```python
from build123d import *

# Parameters (mm, degrees)
F0_W     = 30
F0_H     = 60
F1_DEPTH = 5
F2_R     = 2.196128
F3_DEPTH = 3
F4_R     = 1.034036
F5_DEPTH = 1


with BuildPart() as f1:
    # F0 (on Front) → F1 (new body)
    with BuildSketch(Plane.XZ):
        with Locations((-16.133093, -22.920842)):
            Rectangle(F0_W, F0_H)
    extrude(amount=F1_DEPTH)

    # F2 (on face) → F3 (join)
    with BuildSketch(Plane.XZ.offset(5)):
        with Locations((-7.345827, -21.091014)):
            Circle(F2_R)
    extrude(amount=F3_DEPTH)

    # F4 (on face) → F5 (join)
    with BuildSketch(Plane.XZ.offset(8)):
        with Locations((-7.345827, -21.091014)):
            Circle(F4_R)
    extrude(amount=F5_DEPTH)


solid = f1.part
```
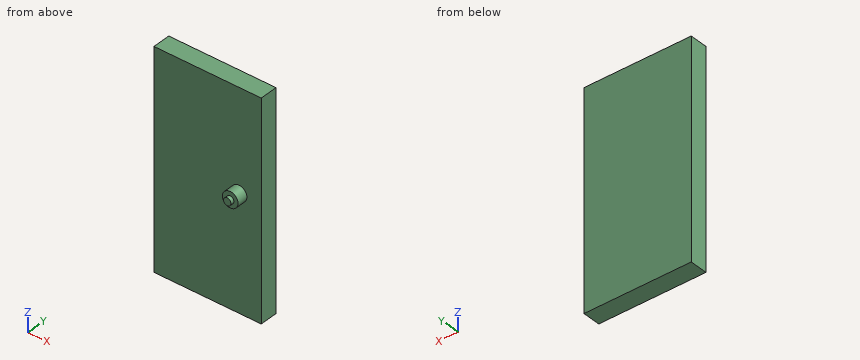
Design review of the part built by this model. Coordinates are the model's own, in mm. Give positions to 0.01 mm unless a question says otherwise; leave off trailing zeros. Loops run counter-clockwise (first coordinate to the right, second up) from the corner with the lowest first, then second, coordinate; pieces in that order, holes last. Notation, with made-up numbers: (47.25, 36.25) -> (78.25, 36.25) arc R18 cw to (78.25, 60.25) -> close; hole circle Ø7 at (-19, -12.5). An arc over 180 degrees is marked (long way). Write each question's results on one line, items separated by ' | '.
Q1. Take a section at C-C, the plane y = -6.75. Write out the cut boundary in (x, z).
Reply:
outline: circle Ø4.39 at (-7.35, -21.09)
Q2. Take a section at A-A, the plane z = -5. Write out the cut boundary in (x, y).
Reply:
outline: (-31.13, -5) -> (-1.13, -5) -> (-1.13, 0) -> (-31.13, 0) -> close
Q3. Wall thickness on L1, parallel to Y at x = -20.5, z = -43: over which ranges is the line inside the solid? List them lowest first.
Reply:
L1: y = -5 to 0
Q4. Take a section at B-B, the plane x = -13.5. Write out the cut boundary in (y, z), plus the area to 3 significant figures.
Reply:
outline: (-5, -52.92) -> (0, -52.92) -> (0, 7.08) -> (-5, 7.08) -> close | area: 300 mm²
Q5. For pin 1 Ø5 at (x, z) = (-23.5, -33.5) entering from +Y; pin 2 Ø12 at (x, z) = (-13, -36.5) entering from -Y, all flat-tipped, find the tip position at first contact; note any pin that passes through.
Reply:
pin 1: stops at y = 0 | pin 2: stops at y = -5
